```python
from build123d import *

# Parameters (mm, degrees)
F1_DEPTH = 30


with BuildPart() as f1:
    # F0 (on Front) → F1 (new body)
    with BuildSketch(Plane.XZ):
        with BuildLine():
            Line((0, 70), (0, 0))
            Line((0, 0), (30, 0))
            Line((30, 0), (30, 20))
            ThreePointArc((30, 20), (40, 30), (50, 20))
            Line((50, 20), (50, 0))
            Line((50, 0), (115, 0))
            Line((115, 0), (115, 20))
            ThreePointArc((115, 20), (125, 30), (135, 20))
            Line((135, 20), (135, 0))
            Line((135, 0), (175, 0))
            Line((175, 0), (175, 44))
            Line((175, 44), (135, 90))
            Line((135, 90), (100, 90))
            Line((100, 90), (100, 60))
            ThreePointArc((100, 60), (85, 45), (70, 60))
            Line((70, 60), (70, 90))
            Line((70, 90), (20, 90))
            ThreePointArc((20, 90), (5.857864, 84.142136), (0, 70))
        make_face()
    extrude(amount=F1_DEPTH)


solid = f1.part
```
Model file for the job. Use its own axes, mm. A direction names the side the tool comes from. Coordinates: 2 decimals unless noted, no trailing zeros. Order: outer loops, then holes, each group sorted by start corner. A loop starts at its lowest first (then second) coordinate and runs counter-clockwise, first axis right, second up. Notation, with made-up numbers: (-24.5, -28.75) -> (30.5, -28.75) arc R12 cw to (30.5, -22.75) -> close; hole circle Ø6 at (23, 4). An arc over 180 degrees is marked (long way). Answer as a JSON object with one key per item and string values. Group by question number.
1) Pull direction X, two halves, no side cores. Call faces 1 (the face through (0, -15, 35)), 2 (the face through (45, -15, 90)), 3 (the face through (100, -15, 75)): +X half, -X half, draft (parallel to the pull), parting line (faces both ways), or undercut.
2) Cut at C-C, the plane x = 125. Write the cut outline in (y, z), then the cut area to 3 significant figures.
3) Which spindle directions (+Z, -Z, +X, -X, +Y, -Y) get a long thin tool onto all of the face, cutting with end or side? Do faces 4 (the face through (70, -15, 75)), 5 (the face through (135, -15, 10)), 6 (the face through (86, -30, 36)). Say none if no direction does.
4) Cut at A-A, the plane y = -2.5. Write the cut outline in (x, z), then the cut area to 3 significant figures.
5) Flat gauge pin, fed straight in: pin 1 (9 mm diameter, centred on y = -12, z = 79.5, fed in from +X). Where does the tip first touch, or does it go through?
6) Cut at D-D, the plane x = 78. Write the cut outline in (y, z).
7) Cut at B-B, the plane z = 24. Write the cut outline in (x, y).
8) Drill centre lines: L1, parallel to X at y = -17, z = 6; L2, parallel to X at y = -15.25, z = 25; L3, parallel to X at y = -28.5, z = 68. Where is each one in solid material? Low to high.
Check values:
{
 "1": {"face 1": "-X half", "face 2": "draft", "face 3": "undercut"},
 "2": {"outline": "(-30, 30) -> (0, 30) -> (0, 90) -> (-30, 90) -> close", "area": "1,800 mm²"},
 "3": {"face 4": "+Z, +Y, -Y", "face 5": "-Z, +Y, -Y", "face 6": "+Z, -Z, +X, -X, -Y"},
 "4": {"outline": "(0, 0) -> (30, 0) -> (30, 20) arc R10 cw to (50, 20) -> (50, 0) -> (115, 0) -> (115, 20) arc R10 cw to (135, 20) -> (135, 0) -> (175, 0) -> (175, 44) -> (135, 90) -> (100, 90) -> (100, 60) arc R15 cw to (70, 60) -> (70, 90) -> (20, 90) arc R20 ccw to (0, 70) -> close", "area": "12,400 mm²"},
 "5": {"pin 1": "stops at x = 148.04"},
 "6": {"outline": "(-30, 0) -> (0, 0) -> (0, 46.73) -> (-30, 46.73) -> close"},
 "7": {"outline": "(0, -30) -> (30.83, -30) -> (30.83, 0) -> (0, 0) -> close; (49.17, -30) -> (115.83, -30) -> (115.83, 0) -> (49.17, 0) -> close; (134.17, -30) -> (175, -30) -> (175, 0) -> (134.17, 0) -> close"},
 "8": {"L1": "x = 0 to 30, 50 to 115, 135 to 175", "L2": "x = 0 to 31.34, 48.66 to 116.34, 133.66 to 175", "L3": "x = 0 to 70, 100 to 154.13"}
}
